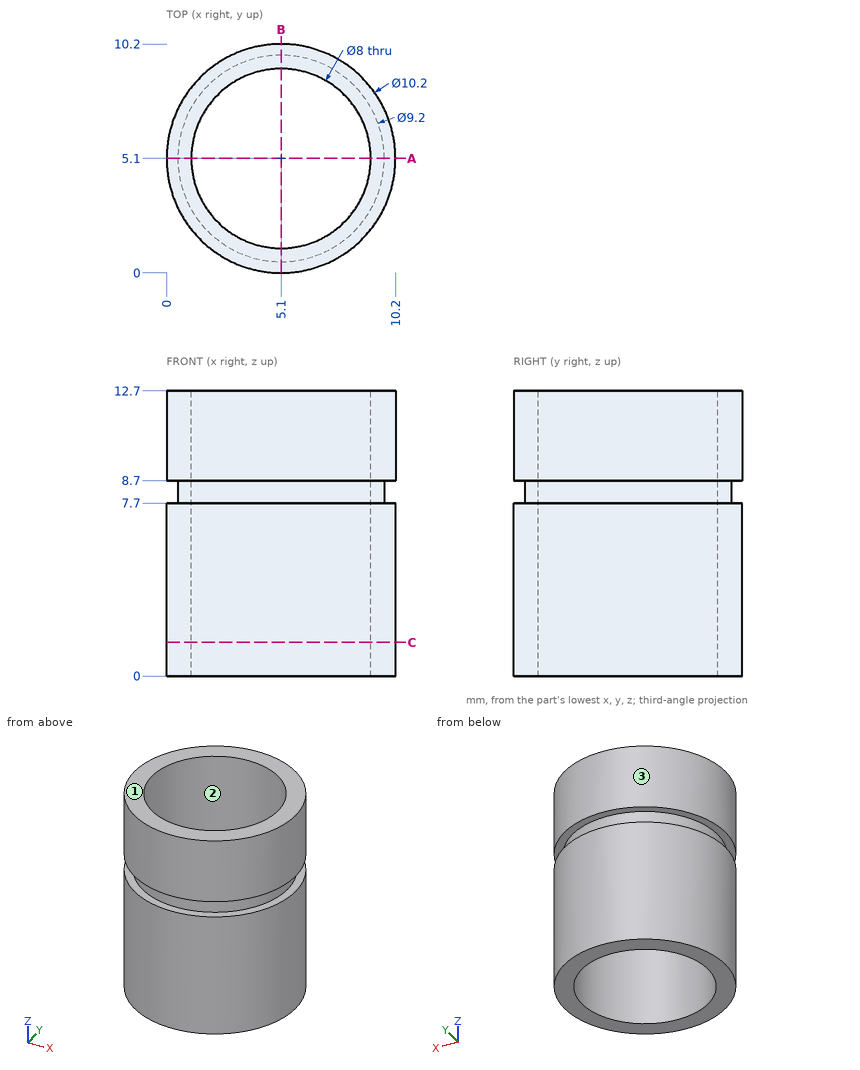
Geometry check sheet. Reference: drawing and pictorial views, mm from the part's lowest x, y, z. Round coordinates to 2 decimals unless told otherwise and drop trailing zeros. Loops run counter-clockwise (first coordinate to the right, second up) from the corner with the lowest first, then second, coordinate; pieces in that order, holes last. Notation, with made-up numbers: (-36.75, 87) -> (13.25, 87) arc R30 cw to (13.25, 122) -> close; hole circle Ø8 at (37, -5). An arc over 180 degrees is marked (long way). Answer as a JSON object with one key per item and string values. Group by question number.
Item 1: Thickness scan on line 1 along Z through (x, y) = (1.75, 8.75); line 2 along Y through (x, z) = (1.75, 8); line 3 along X through (y, z) = (3, 8). Record the ranges inside material, lowest first.
Item 2: Depth check by flat-ended pin: pin 1 Ø1 at (x, z) = (6.5, 3.5) entering from +Y; pin 2 Ø1 at (x, z) = (8, 6) entering from +Y. Enter the tip coordinate at first touch or a pass-through.
Item 3: Release check for a two-part mould opening along Y. For the marked faces 1, 2 and 3 record: pulls with the +Y half, pulls with the -Y half, needs draft (parallel to the pull), parting line crosses it, or undercut.
Item 4: Cross-section at C-C, the plane z = 1.5. Record the cut outline in (x, y), plus the area to 3 significant figures.
Item 5: Cross-section at A-A, the plane y = 5.1. Record the cut outline in (x, z).
Determined:
{
 "1": {"line 1": "z = 0 to 7.7, 8.7 to 12.7", "line 2": "y = 1.95 to 2.91, 7.29 to 8.25", "line 3": "x = 1.01 to 1.7, 8.5 to 9.19"},
 "2": {"pin 1": "stops at y = 10.12", "pin 2": "stops at y = 9.6"},
 "3": {"face 1": "needs draft", "face 2": "undercut", "face 3": "parting line crosses it"},
 "4": {"outline": "circle Ø10.2 at (5.1, 5.1); hole circle Ø8 at (5.1, 5.1)", "area": "31.4 mm²"},
 "5": {"outline": "(0, 0) -> (1.1, 0) -> (1.1, 12.7) -> (0, 12.7) -> (0, 8.7) -> (0.5, 8.7) -> (0.5, 7.7) -> (0, 7.7) -> close; (9.1, 0) -> (10.2, 0) -> (10.2, 7.7) -> (9.7, 7.7) -> (9.7, 8.7) -> (10.2, 8.7) -> (10.2, 12.7) -> (9.1, 12.7) -> close"}
}
